For this review, take the finished solid that the model builds, in its own axes (mm). Face numbers are marked on the shaded views. A direction names the side the tool comes from. Coordinates: 2 decimals unless noted, no trailing zeros. Loops run counter-clockwise (first coordinate to the right, second up) from the corner with the lowest first, then second, coordinate; pieces in that order, holes last. Notation, with made-up numbers: (-2, -16.5) - (14, -16.5) arc R5 cw to (14, -11.5) - close; hole circle Ø3 at (53, 52.25). An arc over 180 degrees is marked (long way). Answer as a JSON object with one key per item and string values. Group by question number.
Item 1: To check wall thickness, follow line 1 (Z direction, x = -8.75, y = -10.5); line 2 (Z direction, x = -4.5, y = -34); line 3 (Y direction, x = -14, z = 4.5). State the ranges of each line that lie inside material, in increasing order.
Item 2: We need section A-A (x = -8). State how many separate pieces and enclosed holes the cut face has, then the cut area to 3 significant figures.
Item 3: We need section D-D (z = 30.5). Give the boundary of the cut face in (x, y).
Item 4: We need section C-C (y = -27). Give the boundary of the cut face in (x, z).
Item 5: We need section B-B (x = -2.5). Give the boundary of the cut face in (y, z), then the cut area to 3 significant figures.
Item 6: Clearance check with flat-ended pins moving along their axes: pin 1 (3 mm diameter, centred on x = -13.5, y = -13.5, fed in from -Z); pin 2 (5 mm diameter, centred on x = -9, z = 49, fed in from +Y); pin 3 (8 mm diameter, centred on x = -4.5, y = -28, fed in from +Z). State where each tip first meets the part, or that it passes through.
Item 7: Tool access review of the marked faces 1, 2, 3 and 4: name each direction out of +Z, -Z, +X, -X, +Y, -Y from which nothing blocks a thin tool from reaching the whole face with its end or side.
from build123d import *

# Parameters (mm, degrees)
SKETCH1_R           = 4
BOSS_EXTRUDE1_DEPTH = 16
SKETCH2_R           = 2
CUT_EXTRUDE1_DEPTH  = 77.491311533
SKETCH3_R           = 1.5
CUT_EXTRUDE2_DEPTH  = 75.439040429


with BuildPart() as part:
    # Sketch1 → Boss-Extrude1 (new body)
    with BuildSketch(Plane(origin=(0, 0, 0), x_dir=(0, 0, -1), z_dir=(1, 0, 0))):
        with BuildLine():
            Line((-10.309088451, -58.789851982), (-58.982376521, -58.789851982))
            Line((-58.982376521, -58.789851982), (-58.982376521, -48.789851982))
            Line((-58.982376521, -48.789851982), (-18.982376521, -48.789851982))
            Line((-18.982376521, -48.789851982), (-8.982376521, -38.789851982))
            Line((-8.982376521, -38.789851982), (-8.982376521, -10.789851982))
            ThreePointArc((-8.982376521, -10.789851982), (-0.982376521, -2.789851982), (7.017623479, -10.789851982))
            Line((7.017623479, -10.789851982), (7.017623479, -45.289851982))
            Line((7.017623479, -45.289851982), (17.017623479, -45.289851982))
            Line((17.017623479, -45.289851982), (17.017623479, -48.289851982))
            Line((17.017623479, -48.289851982), (7.017623479, -48.289851982))
            Line((7.017623479, -48.289851982), (7.017623479, -50.789851982))
            ThreePointArc((7.017623479, -50.789851982), (6.916823965, -52.055802887), (6.616965556, -53.289851982))
            Line((6.616965556, -53.289851982), (17.017623479, -53.289851982))
            Line((17.017623479, -53.289851982), (17.017623479, -56.289851982))
            Line((17.017623479, -56.289851982), (4.827098499, -56.289851982))
            ThreePointArc((4.827098499, -56.289851982), (2.179901139, -58.138321211), (-0.982376521, -58.789851982))
            Line((-0.982376521, -58.789851982), (-10.309088451, -58.789851982))
        make_face()
        with Locations((-0.982376521, -10.789851982)):
            Circle(SKETCH1_R, mode=Mode.SUBTRACT)
        with Locations((-0.982376521, -50.789851982)):
            Circle(SKETCH1_R, mode=Mode.SUBTRACT)
    extrude(amount=-BOSS_EXTRUDE1_DEPTH)

    # Sketch2 → Cut-Extrude1 (cut, through all)
    with BuildSketch(Plane(origin=(0, -48.789851982, 0), x_dir=(1, 0, 0), z_dir=(0, 1, 0))):
        with Locations(Location((-8, -43.982376521, 0), (0, 0, 270))):
            Circle(SKETCH2_R)
    extrude(amount=-CUT_EXTRUDE1_DEPTH, mode=Mode.SUBTRACT)

    # Sketch3 → Cut-Extrude2 (cut, through all)
    with BuildSketch(Plane(origin=(0, -45.289851982, 0), x_dir=(1, 0, 0), z_dir=(0, 1, 0))):
        with Locations(Location((-8, 12.017623479, 0), (0, 0, 270))):
            Circle(SKETCH3_R)
    extrude(amount=-CUT_EXTRUDE2_DEPTH, mode=Mode.SUBTRACT)


solid = part.part
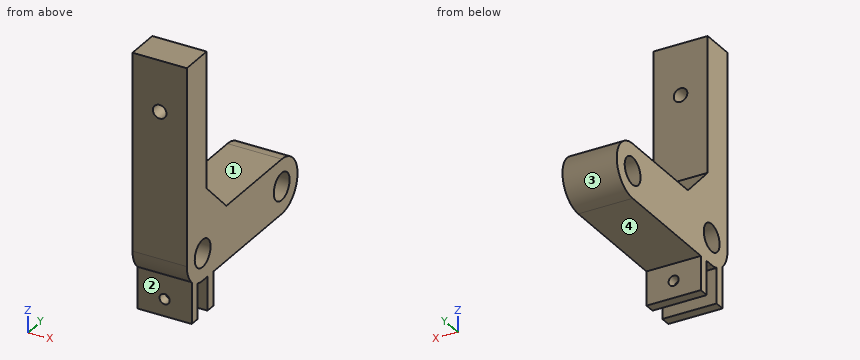
Check sheet entries:
{
 "1": {"line 1": "z = -7.01 to -3.01, 4.97 to 8.98", "line 2": "z = -7.02 to 8.98", "line 3": "y = -58.79 to -52.69, -48.89 to -12.69, -8.89 to -3.6"},
 "2": {"separate pieces": "4", "enclosed holes": "2", "area": "1,310 mm2"},
 "3": {"outline": "(-16, -58.79) - (0, -58.79) - (0, -48.79) - (-16, -48.79) - close"},
 "4": {"outline": "(-16, -7.02) - (0, -7.02) - (0, 8.98) - (-16, 8.98) - close"},
 "5": {"outline": "(-58.79, 0.98) arc R8 ccw to (-56.29, -4.83) - (-56.29, -17.02) - (-53.29, -17.02) - (-53.29, -6.62) arc R8 ccw to (-50.79, -7.02) - (-48.29, -7.02) - (-48.29, -17.02) - (-45.29, -17.02) - (-45.29, -7.02) - (-10.79, -7.02) arc R8 ccw to (-10.79, 8.98) - (-38.79, 8.98) - (-48.79, 18.98) - (-48.79, 58.98) - (-58.79, 58.98) - close; hole circle Ø8 at (-50.79, 0.98); hole circle Ø8 at (-10.79, 0.98)", "area": "1,370 mm2"},
 "6": {"pin 1": "stops at z = -7.02", "pin 2": "stops at y = -48.79", "pin 3": "stops at z = 8.98"},
 "7": {"face 1": "+Z, +X, -X, +Y", "face 2": "-Z, +X, -X, -Y", "face 3": "+X, -X, +Y", "face 4": "-Z, +X, -X, +Y"}
}
